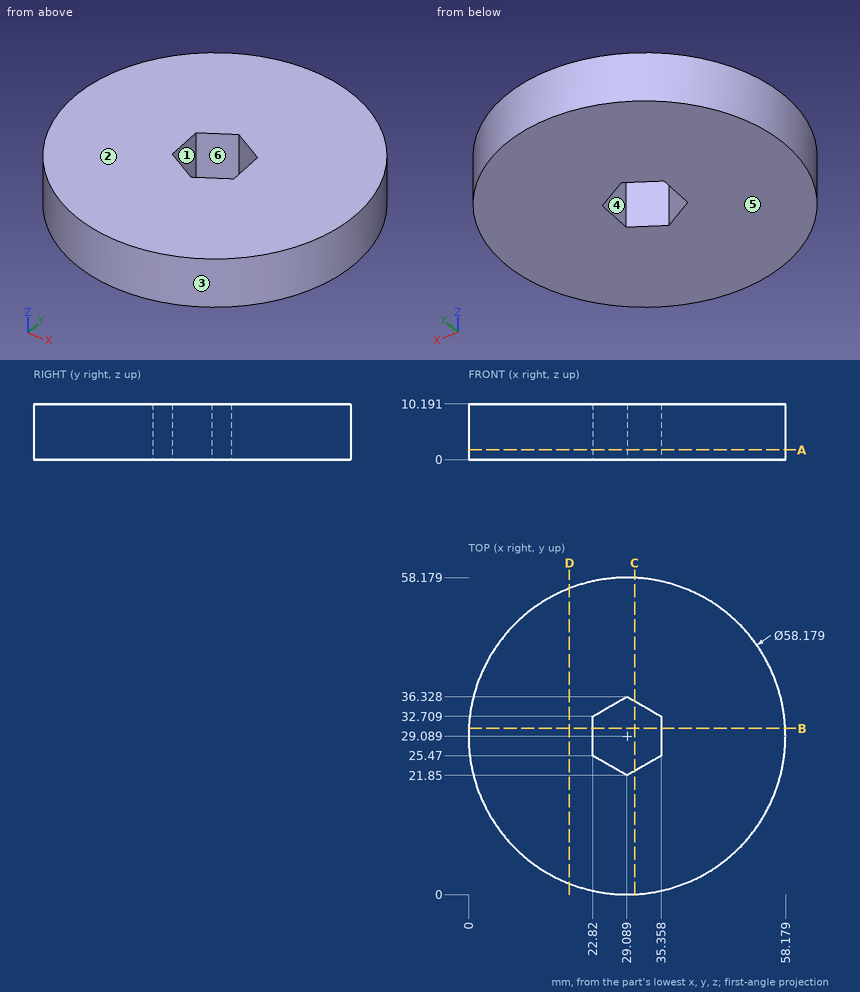
Here's the drawing with two shaded views (mm, measured from the low corner). I have some questions. A direction names the side the tool comes from. Give positions to 0.01 mm unless a question says otherwise; leave off trailing zeros. Order: outer loops, then holes, each group sorted by start corner. A loop starts at its lowest first (then second) coordinate and runs counter-clockwise, first axis right, second up. Notation, with made-up numbers: (60.25, 21.5) - (76.25, 21.5) arc R14 cw to (76.25, 26.5) - close; hole circle Ø10 at (72.5, 3). An arc over 180 degrees is marked (long way). Write each question's results on one line, items separated by ' | '.
1) Suppose I cut it at C-C, the plane x = 30.5. Write out the boundary of the cut face in (y, z) (1 decimal).
Final values:
outline: (0, 0) - (22.7, 0) - (22.7, 10.2) - (0, 10.2) - close; (35.5, 0) - (58.1, 0) - (58.1, 10.2) - (35.5, 10.2) - close
2) Suppose I cut it at D-D, the plane x = 18.5. Write out the boundary of the cut face in (y, z) (1 decimal).
Final values:
outline: (2, 0) - (56.2, 0) - (56.2, 10.2) - (2, 10.2) - close
3) Please list where these lines run through material, in increasing order: line 1 along X through (y, z) = (25, 4.5) (1 decimal); line 2 along Y through (x, z) = (25, 1.75); line 3 along X through (y, z) = (25.5, 5.5). Write a range as [from, to].
Final values:
line 1: x = [0.3, 23.6], [34.5, 57.9] | line 2: y = [0.29, 24.21], [33.97, 57.89] | line 3: x = [0.22, 22.82], [35.36, 57.96]
4) On a 3-axis mill with a long thin cutter (end or side, diameter ignored), from which of +Z, -Z, +X, -X, +Y, -Y can I reach the whole of each face in a straight line? I mean the marked faces 1 and 2. Say none if no direction works.
Final values:
face 1: +Z, -Z | face 2: +Z, +X, -X, +Y, -Y
5) Suppose I cut it at A-A, the plane z = 1.75. Write out the boundary of the cut face in (x, y).
Final values:
outline: circle Ø58.18 at (29.09, 29.09); hole (22.82, 25.47) - (29.09, 21.85) - (35.36, 25.47) - (35.36, 32.71) - (29.09, 36.33) - (22.82, 32.71) - close
6) If we mould it in two halves opening along X, with no side actions, what happens to the marked faces 3, 4, 5 and 6? For each: pulls with the +X half, pulls with the -X half, needs draft (parallel to the pull), parting line crosses it, or undercut.
Final values:
face 3: parting line crosses it | face 4: undercut | face 5: needs draft | face 6: undercut
7) Suppose I cut it at B-B, the plane y = 30.5. Write out the boundary of the cut face in (x, z) (1 decimal).
Final values:
outline: (0, 0) - (22.8, 0) - (22.8, 10.2) - (0, 10.2) - close; (35.4, 0) - (58.1, 0) - (58.1, 10.2) - (35.4, 10.2) - close
8) I'm going to push flat-ended pins straight in: pin 1 Ø6 at (x, y) = (17, 27.5) entering from -Z; pin 2 Ø5 at (x, z) = (40, 2) entering from -Y; pin 3 Ø2 at (y, z) = (38, 8.5) entering from -X; pin 4 Ø1 at (y, z) = (20.5, 4) entering from +X. Where does each tip first touch, or does it pass through?
Final values:
pin 1: stops at z = 0 | pin 2: stops at y = 1.24 | pin 3: stops at x = 1.1 | pin 4: stops at x = 57.03
